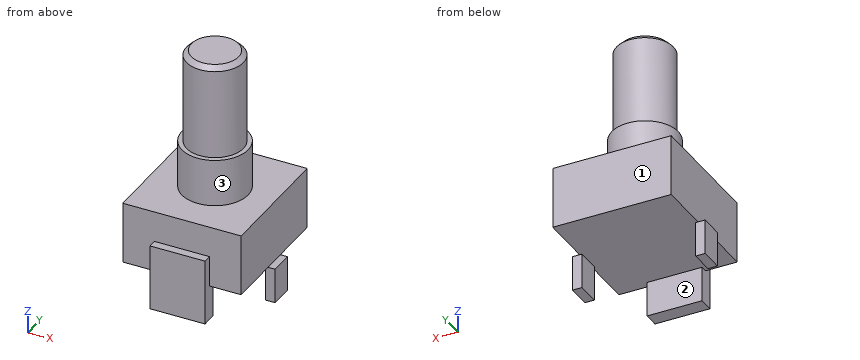
```python
from build123d import *

# Parameters (mm, degrees)
F3_DEPTH       = 6.5
F1_R           = 3.5
F4_DEPTH       = 11.5
F2_R           = 3
F5_DEPTH       = 21.5
F6_SIZE        = 0.5
F7_W           = 1
F7_H           = 2.5
F8_DEPTH       = 3.7
F9_W           = 5.8
F9_H           = 1.6
F10_DEPTH      = 3.25
F10_DEPTH_BACK = 3.7


with BuildPart() as f3:
    # F0 (on Top) → F3 (new body)
    with BuildSketch(Plane.XY):
        Polygon((0, 11.7), (-6.25, 11.7), (-6.25, -1.7), (6.25, -1.7), (6.25, 5), (6.25, 11.7), align=None)
    extrude(amount=F3_DEPTH)

    # F1 (on Top) → F4 (join)
    with BuildSketch(Plane.XY):
        with Locations((0, 5)):
            Circle(F1_R)
    extrude(amount=F4_DEPTH)

    # F2 (on Top) → F5 (join)
    with BuildSketch(Plane.XY):
        with Locations((0, 5)):
            Circle(F2_R)
    extrude(amount=F5_DEPTH)

    # F6
    f6_edges = [f3.edges().sort_by_distance(p)[0] for p in [
        (-3, 5, 21.5),
    ]]
    chamfer(f6_edges, length=F6_SIZE)

    # F7 (on Top) → F8 (join)
    with BuildSketch(Plane.XY):
        with Locations((-6.5, 5)):
            Rectangle(F7_W, F7_H)
        with Locations((6.5, 5)):
            Rectangle(F7_W, F7_H)
    extrude(amount=-F8_DEPTH)

    # F9 (on Top) → F10 (join, two sides)
    with BuildSketch(Plane.XY) as f10_sk:
        with Locations((0, -1.8)):
            Rectangle(F9_W, F9_H)
    extrude(amount=F10_DEPTH)
    extrude(f10_sk.sketch, amount=-F10_DEPTH_BACK)


solid = f3.part
```
Geometry check sheet. Reference: the model listing, model coordinates, mm. Face numbers are marked on the shaded views. A direction names the side the tool comes from. Coordinates: 2 decimals unless noted, no trailing zeros. Loops run counter-clockwise (first coordinate to the right, second up) from the corner with the lowest first, then second, coordinate; pieces in that order, holes last.
Item 1: Access from +Z, -Z, +X, -X, +Y, -Y to the whole of each face (thin tool, end or side, straight path). Record for the marked faces 1, 2 and 3.
Item 2: Sectioned sample at B-B, the plane x = 0. Record the boundary of the cut face in (y, z), then the cut area to 3 significant figures.
Item 3: Sectioned sample at D-D, the plane y = 9.25. Record the boundary of the cut face in (x, z).
Item 4: Sectioned sample at A-A, the plane y = 5. Record the boundary of the cut face in (x, z).
Item 5: Thickness scan on line 1 (Z direction, x = -2.25, y = 7.75); line 2 (X direction, y = 10.25, z = 6); line 3 (Z direction, x = 0.25, y = 4.75). Record the ranges inside material, lowest first.
Item 6: Sectioned sample at C-C, the plane z = 19. Record the boundary of the cut face in (x, y), then the cut area to 3 significant figures.
Item 7: Go/stop test with flat-tipped pins: pin 1 Ø5 at (y, z) = (2.5, 3.5) entering from -X; pin 2 Ø0.8 at (x, z) = (-6.5, -2.5) entering from -Y; pin 3 Ø0.6 at (x, y) = (-6.5, 5) entering from +Z. Record where each tip stops, or that it passes through.
Check result:
1. face 1: +Z, -Z, +X, -X, +Y
1. face 2: -Z, +X, -X, +Y
1. face 3: +Z
2. outline: (-2.6, -3.7) - (-1, -3.7) - (-1, 0) - (11.7, 0) - (11.7, 6.5) - (8.5, 6.5) - (8.5, 11.5) - (8, 11.5) - (8, 21) - (7.5, 21.5) - (2.5, 21.5) - (2, 21) - (2, 11.5) - (1.5, 11.5) - (1.5, 6.5) - (-1.7, 6.5) - (-1.7, 3.25) - (-2.6, 3.25) - close
2. area: 191 mm2
3. outline: (-6.25, 0) - (6.25, 0) - (6.25, 6.5) - (-6.25, 6.5) - close
4. outline: (-7, -3.7) - (-6, -3.7) - (-6, 0) - (6, 0) - (6, -3.7) - (7, -3.7) - (7, 0) - (6.25, 0) - (6.25, 6.5) - (3.5, 6.5) - (3.5, 11.5) - (3, 11.5) - (3, 21) - (2.5, 21.5) - (-2.5, 21.5) - (-3, 21) - (-3, 11.5) - (-3.5, 11.5) - (-3.5, 6.5) - (-6.25, 6.5) - (-6.25, 0) - (-7, 0) - close
5. line 1: z = 0 to 6.5
5. line 2: x = -6.25 to 6.25
5. line 3: z = 0 to 21.5
6. outline: circle Ø6 at (0, 5)
6. area: 28.3 mm2
7. pin 1: stops at x = -6.25
7. pin 2: stops at y = 3.75
7. pin 3: stops at z = 6.5
